from build123d import *

# Parameters (mm, degrees)
SKETCH1_W             = 4
SKETCH1_H             = 66
BOSS_EXTRUDE1_DEPTH   = 1
SKETCH1_2_W           = 4
SKETCH1_2_H           = 66
BOSS_EXTRUDE2_DEPTH   = 1.36844839
SKETCH4_W             = 2
SKETCH4_H             = 66.494663906
BOSS_EXTRUDE3_DEPTH   = 5
SKETCH4_2_W           = 2
SKETCH4_2_H           = 66.494663906
BOSS_EXTRUDE4_DEPTH   = 6.842238407
F_3_0MM_DOWEL_HOLE1_D = 3


with BuildPart() as part:
    # Sketch1 → Boss-Extrude1 (new, along a direction that is not the sketch's normal)
    with BuildSketch(Plane.XY):
        Rectangle(SKETCH1_W, SKETCH1_H)
    extrude(amount=BOSS_EXTRUDE1_DEPTH, dir=(0, 0.6347305132022716, 0.7727335734973478))

    # Sketch1<2> → Boss-Extrude2 (add, along a direction that is not the sketch's normal)
    with BuildSketch(Plane.XY):
        Rectangle(SKETCH1_2_W, SKETCH1_2_H)
    extrude(amount=BOSS_EXTRUDE2_DEPTH, dir=(0, 0.8253106586930028, 0.5646789500660725))

    # Sketch4 → Boss-Extrude3 (add, along a direction that is not the sketch's normal)
    with BuildSketch(Plane.XY.offset(0.772733573)):
        with Locations((0, 0.882062466)):
            Rectangle(SKETCH4_W, SKETCH4_H)
    extrude(amount=BOSS_EXTRUDE3_DEPTH, dir=(0, 0.6347305132022716, 0.7727335734973478))

    # Sketch4<2> → Boss-Extrude4 (add, along a direction that is not the sketch's normal)
    with BuildSketch(Plane.XY.offset(0.772733573)):
        with Locations((0, 0.882062466)):
            Rectangle(SKETCH4_2_W, SKETCH4_2_H)
    extrude(amount=BOSS_EXTRUDE4_DEPTH, dir=(0, 0.8253106586930028, 0.5646789500660725))

    # Ø3.0mm Dowel Hole1 (through all)
    with Locations(Plane.ZY.offset(1)):
        with Locations((2.704567507, -14.191616921), (2.704567507, 15.808383079)):
            Hole(F_3_0MM_DOWEL_HOLE1_D / 2)


solid = part.part
Check sheet for the modelled part. Datum: model origin and axes. Units: mm. A direction names the side the tool comes from. Round coordinates to 2 decimals unless told otherwise and drop trailing zeros. Order: outer loops, then holes, each group sorted by start corner. A loop starts at its lowest first (then second) coordinate and runs counter-clockwise, first axis right, second up. Notation, with made-up numbers: M 35.5,83 L 58.5,83 A24 ccw 58.5,98 Z; hole C 68.5,-18 d5. An arc over 180 degrees is marked long. One line per item, written item: value. Start each with the question number.
1. Gauge pin test, flat ends, axial feed: P1, Ø1.2, axis at y = -3.5, z = 2, coming from the -X side; P2, Ø0.5, axis at x = -1.5, y = -32, coming from the +Z side. Record the tip position at first contact, or that the pin passes through.
2. Release check for a two-part mould opening along Y. For faces 3 (the flat face through (-1, 3, 3)), 4 (the cylindrical face through (0.014, -12.704, 2.9)), 5 (the flat face through (-0.028, -31.546, 1.771)) record: released by +Y, released by -Y, zero draft, split by the parting line, or undercut.
3. Access from +Z, -Z, +X, -X, +Y, -Y to the whole of each face (thin tool, end or side, straight path). Record for faces 1 (the flat face through (1, 3, 3)), 2 (the cylindrical face through (0.014, 17.296, 2.9)).
4. Section check C-C on x = -0.4. Enter the section's corners in (y, z), and give its area (3 significant figures).
5. Section check D-D on y = 0.5. Enter the section's corners in (x, z), and give its area (3 significant figures).
6. Scan lines: line 1 along Y through (x, z) = (0.1, 2.9); line 2 along Y through (x, z) = (0.1, 1.55); line 3 along X through (y, z) = (0.5, 3.2). Record each from-to range of solid material in increasing order.
7. Section check A-A on z = 3.25. Enter the section's corners in (x, y).
8. Section check B-B on y = -13.5. Enter the section's corners in (x, z), and give its area (3 significant figures).
Results found:
1. P1: x = -1
1. P2: z = 0.77
2. face 3: zero draft
2. face 4: undercut
2. face 5: released by -Y
3. face 1: +Z, +X, +Y, -Y
3. face 2: +X, -X
4. outline: M -33,0 L 33,0 L 39.78,4.64 L -29.19,4.64 Z; hole C -14.19,2.7 d3; hole C 15.81,2.7 d3
4. area: 299 mm^2
5. outline: M -2,0 L 2,0 L 2,0.77 L 1,0.77 L 1,4.64 L -1,4.64 L -1,0.77 L -2,0.77 Z
5. area: 10.8 mm^2
6. line 1: -30.62 to -15.68, -12.7 to 14.32, 17.3 to 37.24
6. line 2: -31.73 to -15.15, -13.23 to 14.85, 16.77 to 35.27
6. line 3: -1 to 1
7. outline: M -1,-30.33 L 1,-30.33 L 1,-15.59 L -1,-15.59 Z; M -1,-12.79 L 1,-12.79 L 1,14.41 L -1,14.41 Z; M -1,17.21 L 1,17.21 L 1,37.75 L -1,37.75 Z
8. outline: M -2,0 L 2,0 L 2,0.77 L 1,0.77 L 1,1.37 L -1,1.37 L -1,0.77 L -2,0.77 Z; M -1,4.04 L 1,4.04 L 1,4.64 L -1,4.64 Z
8. area: 5.49 mm^2
